Here's how the part is built. I have some questions about the finished solid (model axes, mm). Round coordinates to 2 decimals unless told otherwise and drop trailing zeros. Order: outer loops, then holes, each group sorted by start corner. A loop starts at its lowest first (then second) coordinate and runs counter-clockwise, first axis right, second up.
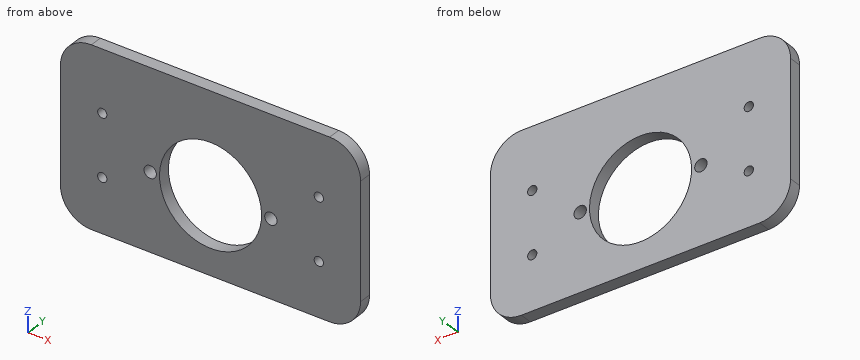
```python
from build123d import *

# Parameters (mm, degrees)
SKETCH_1_W          = 97
SKETCH_1_H          = 57.5
SKETCH_1_R          = 16.5
SKETCH_1_R_2        = 2
EXTRUDE_1_DEPTH     = 4
FILLET_1_R          = 10
SKETCH_2_R          = 1.5
CUT_EXTRUDE_1_DEPTH = 10


with BuildPart() as part:
    # Эскиз1 → Бобышка-Вытянуть1 (new body)
    with BuildSketch(Plane(origin=(0, 0, 0), x_dir=(1, 0, 0), z_dir=(0, 1, 0))):
        with Locations((48.5, 28.75)):
            Rectangle(SKETCH_1_W, SKETCH_1_H)
        with Locations(Location((48.5, 32.5, 0), (0, 0, 270))):
            Circle(SKETCH_1_R, mode=Mode.SUBTRACT)
        with Locations(Location((29, 32.5, 0), (0, 0, 270))):
            Circle(SKETCH_1_R_2, mode=Mode.SUBTRACT)
        with Locations(Location((68, 32.5, 0), (0, 0, 90))):
            Circle(SKETCH_1_R_2, mode=Mode.SUBTRACT)
    extrude(amount=EXTRUDE_1_DEPTH)

    # Скругление1
    fillet_1_edges = [part.edges().sort_by_distance(p)[0] for p in [
        (0, 2, -57.5),
        (97, 2, -57.5),
        (97, 2, 0),
        (0, 2, 0),
    ]]
    fillet(fillet_1_edges, radius=FILLET_1_R)

    # Эскиз2 → Вырез-Вытянуть1 (cut)
    with BuildSketch(Plane(origin=(0, 4, 0), x_dir=(1, 0, 0), z_dir=(0, 1, 0))):
        with Locations(Location((13.5, 20, 0), (0, 0, 270))):
            Circle(SKETCH_2_R)
        with Locations(Location((13.5, 40, 0), (0, 0, 270))):
            Circle(SKETCH_2_R)
        with Locations(Location((83.5, 40, 0), (0, 0, 90))):
            Circle(SKETCH_2_R)
        with Locations(Location((83.5, 20, 0), (0, 0, 90))):
            Circle(SKETCH_2_R)
    extrude(amount=-CUT_EXTRUDE_1_DEPTH, mode=Mode.SUBTRACT)


solid = part.part
```
1. If we section it at C-C, the plane y = 1.5: Write out the boundary of the cut face in (x, z).
Evaluation:
outline: (0, -47.5) arc R10 ccw to (10, -57.5) - (87, -57.5) arc R10 ccw to (97, -47.5) - (97, -10) arc R10 ccw to (87, 0) - (10, 0) arc R10 ccw to (0, -10) - close; hole circle Ø3 at (13.5, -40); hole circle Ø3 at (13.5, -20); hole circle Ø4 at (29, -32.5); hole circle Ø33 at (48.5, -32.5); hole circle Ø4 at (68, -32.5); hole circle Ø3 at (83.5, -40); hole circle Ø3 at (83.5, -20)
2. I need wall thicknesses on probe 1 along X at (y, z) = (2.5, -32.5); probe 2 along Z at (x, y) = (83.5, 2.85); probe 3 along X at (y, z) = (1.9, -19). Which ranges of each line are inside material? Lowest first, please.
Evaluation:
probe 1: x = 0 to 27, 31 to 32, 65 to 66, 70 to 97
probe 2: z = -57.5 to -41.5, -38.5 to -21.5, -18.5 to 0
probe 3: x = 0 to 12.38, 14.62 to 39.01, 57.99 to 82.38, 84.62 to 97
3. If we section it at D-D, the plane z = -40: Write out the boundary of the cut face in (x, y).
Evaluation:
outline: (0, 0) - (12, 0) - (12, 4) - (0, 4) - close; (15, 0) - (33.8, 0) - (33.8, 4) - (15, 4) - close; (63.2, 0) - (82, 0) - (82, 4) - (63.2, 4) - close; (85, 0) - (97, 0) - (97, 4) - (85, 4) - close
4. If we section it at A-A, the plane x = 83.5: Write out the boundary of the cut face in (y, z).
Evaluation:
outline: (0, -57.5) - (4, -57.5) - (4, -41.5) - (0, -41.5) - close; (0, -38.5) - (4, -38.5) - (4, -21.5) - (0, -21.5) - close; (0, -18.5) - (4, -18.5) - (4, 0) - (0, 0) - close
5. If we section it at B-B, the plane x = 29: Write out the boundary of the cut face in (y, z), and give its area (3 significant figures).
Evaluation:
outline: (0, -57.5) - (4, -57.5) - (4, -34.5) - (0, -34.5) - close; (0, -30.5) - (4, -30.5) - (4, 0) - (0, 0) - close
area: 214 mm2
